Build history of the part. All positions in model axes, mm. A direction names the side the tool comes from. Round coordinates to 2 decimals unless told otherwise and drop trailing zeros. Answer as a JSON object with one key per item and string values. Group by question number.
Item 1: Flat gauge pins, fed straight in: pin 1 (0.6 mm diameter, centred on x = 27, z = 1, fed in from +Y); pin 2 (0.6 mm diameter, centred on x = 0, z = 1, fed in from -Y). Where does each tip first touch, or does it go through?
Item 2: Which spindle directions (+Z, -Z, +X, -X, +Y, -Y) get a long thin tool onto all of the face, cutting with end or side? Do faces 4 (the flat face through (-7, 9.45, 1)), 5 (the flat face through (27, 1.447, 1)), 6 (the flat face through (27, 5.994, 1)). Say none if no direction does.
Item 3: Two-plate mould, pull along Z, no slides. Class faces 1 (the flat face through (-1, 5, 1.2)), 2 (the flat face through (-1, 5, 0)), 3 (the flat face through (-7, 0, 1)): +Z half, -Z half, draft (parallel to the pull), parting line (faces both ways), or undercut.
Item 4: Probe line 1 (Y direction, x = -8, z = 1.15); line 2 (X direction, y = 6.75, z = 0.45); line 3 (X direction, y = 8.25, z = 0.85). List the from-to ranges inside material, lowest first. Write a range as from..to.
from build123d import *

# Parameters (mm, degrees)
F1_DEPTH = 1.2


with BuildPart() as f1:
    # F0 (on Top) → F1 (new body)
    with BuildSketch(Plane.XY):
        with BuildLine():
            Line((-31.6033400595, 0), (-18.3987915516, 0))
            Line((-18.3987915516, 0), (17.361568287, 0))
            add(Edge.make_bspline(
                [(17.361568287, 0), (17.6653276456, -0.0151373092), (18.5618703821, 0.0351687115), (19.4891966539, 0.7192725546), (19.8618906847, 1.5062680295), (22.6219379208, 1.4758684176), (23.2729754299, 1.4467175351)],
                knots=[0, 0, 0, 0, 0.223860151, 0.4395498979, 0.6269841693, 1, 1, 1, 1], degree=3))
            Line((23.2729754299, 1.4467175351), (30.3966599405, 1.4467175351))
            Line((30.3966599405, 1.4467175351), (30.3966599405, 5.9939725325))
            Line((30.3966599405, 5.9939725325), (22.6935977936, 5.9939725325))
            add(Edge.make_bspline(
                [(15.9988217056, 9.45), (16.4529830217, 9.4699785113), (17.3664699522, 8.7071065894), (18.9562119726, 6.8036674365), (19.5039672266, 5.8425249718), (22.1805847091, 5.9939725325), (22.6935977936, 5.9939725325)],
                knots=[0, 0, 0, 0, 0.2210198142, 0.5029222248, 0.6921587786, 1, 1, 1, 1], degree=3))
            Line((15.9988217056, 9.45), (-31.6033400595, 9.45))
            Line((-31.6033400595, 9.45), (-31.6033400595, 0))
        make_face()
    extrude(amount=F1_DEPTH)


solid = f1.part
Geometry says:
{
 "1": {"pin 1": "stops at y = 5.99", "pin 2": "stops at y = 0"},
 "2": {"face 4": "+Z, -Z, +X, -X, +Y", "face 5": "+Z, -Z, +X, -Y", "face 6": "+Z, -Z, +X, +Y"},
 "3": {"face 1": "+Z half", "face 2": "-Z half", "face 3": "draft"},
 "4": {"line 1": "y = 0..9.45", "line 2": "x = -31.6..18.94", "line 3": "x = -31.6..17.71"}
}
